from build123d import *

# Parameters (mm, degrees)
SKETCH_1_R          = 1
EXTRUDE_1_DEPTH     = 10.5
SKETCH_2_W          = 9.3
SKETCH_2_H          = 27
CUT_EXTRUDE_1_DEPTH = 10.5
FILLET_1_R          = 4
FILLET_2_R          = 0.3
SKETCH_3_R          = 1.25
CUT_EXTRUDE_2_DEPTH = 19


with BuildPart() as part:
    # 草图1 → 凸台-拉伸1 (new body)
    with BuildSketch(Plane.XY):
        with BuildLine():
            ThreePointArc((7, 0), (4, 3), (1, 0))
            Line((1, 0), (1, -1))
            Line((1, -1), (0, -1))
            Line((0, -1), (0, -21.5))
            add(Edge.make_bspline(
                [(0, -21.5), (0, -22.851375424), (-0.954237794, -23.948160578)],
                knots=[0, 0, 0, 0.976850958, 0.976850958, 0.976850958], degree=2))
            add(Edge.make_bspline(
                [(7, 0), (7, -3.461774358), (6.888539552, -11.820950193), (2.535059444, -19.986776398), (-0.954237794, -23.948160578)],
                knots=[0, 0, 0, 0, 0.379767853, 0.997303013, 0.997303013, 0.997303013, 0.997303013], degree=3))
        make_face()
        with Locations(Location((4, 0, 0), (0, 0, 180))):
            Circle(SKETCH_1_R, mode=Mode.SUBTRACT)
    extrude(amount=EXTRUDE_1_DEPTH)

    # 草图2 → 切除-拉伸1 (cut)
    with BuildSketch(Plane.ZY.offset(-0.6)):
        with Locations((5.25, -10.44816051)):
            Rectangle(SKETCH_2_W, SKETCH_2_H)
    extrude(amount=-CUT_EXTRUDE_1_DEPTH, mode=Mode.SUBTRACT)

    # 圆角1
    fillet_1_edges = [part.edges().sort_by_distance(p)[0] for p in [
        (0.6, -22.041590232, 5.25),
    ]]
    fillet(fillet_1_edges, radius=FILLET_1_R)

    # 圆角2
    fillet_2_edges = [part.edges().sort_by_distance(p)[0] for p in [
        (0, -11.25, 10.5),
        (-0.248254444, -22.812327553, 0),
        (0, -11.25, 0),
        (1, -1, 10.2),
        (-0.248254444, -22.812327553, 10.5),
        (1, -1, 0.3),
    ]]
    fillet(fillet_2_edges, radius=FILLET_2_R)

    # 草图3 → 切除-拉伸2 (cut)
    with BuildSketch(Plane(origin=(0, 0, 0), x_dir=(-1, 0, 0), z_dir=(0, 0, -1))):
        with Locations(Location((-3.2, -8.5, 0), (0, 0, 270))):
            Circle(SKETCH_3_R)
    extrude(amount=-CUT_EXTRUDE_2_DEPTH, mode=Mode.SUBTRACT)


solid = part.part
CAD build for the part. Positions are in the model's coordinates, mm. A direction names the side the tool comes from. Give positions to 0.01 mm unless a question says otherwise; leave off trailing zeros. Answer in a Markdown table with one row per item. Add a question column.
Item 1: Drop flat-ended pins along their axis: P1, Ø0.6, axis at x = 0, z = 7.5, coming from the +Y side; P2, Ø2, axis at x = 3.5, z = 5, coming from the -Y side; P3, Ø1, axis at y = -4.5, z = 8.5, coming from the -X side; P4, Ø3, axis at y = -13.5, z = 3.5, coming from the +X side. Give the stop position or say it passes through.
Item 2: Probe probe 1 along Z at (x, y) = (1.25, -2); probe 2 along Y at (x, z) = (4, 0.25); probe 3 along X at (y, z) = (-13, 2.75). List the from-to ranges inside material, lowest first.
Item 3: Tool access for faces 1 (the face through (0, -11, 5)), 2 (the face through (3, -7, 10.5)), 3 (the face through (0.6, -11, 5)): list every direction of +Z, -Z, +X, -X, +Y, -Y with a clear straight run to the whole face (end or side of a thin tool).
Item 4: Mould opens along Y. For faces 4 (the face through (4.1, 3, 0.3)), 5 (the face through (4, -7, 0.6)), 6 (the face through (4.8, 0.6, 0.3)) say: +Y half, -Y half, draft (parallel to the pull), parting line (faces both ways), or undercut.
Item 5: Band-saw the part on A-A on x = 3.75. Give the number of separate pieces and of enclosed holes in the cut face, then the cut area to 3 significant figures.
Reply:
| question | item | result |
|---|---|---|
| 1 | P1 | stops at y = -1 |
| 1 | P2 | passes through |
| 1 | P3 | stops at x = 0 |
| 1 | P4 | stops at x = 0.6 |
| 2 | probe 1 | z = 0 to 0.6, 9.9 to 10.5 |
| 2 | probe 2 | y = -16.47 to -9.46, -7.54 to -1, 1 to 3 |
| 2 | probe 3 | x = 0 to 0.6 |
| 3 | face 1 | +Z, -Z, -X, +Y |
| 3 | face 2 | +Z, +X, -X, +Y, -Y |
| 3 | face 3 | +X, +Y, -Y |
| 4 | face 4 | +Y half |
| 4 | face 5 | draft |
| 4 | face 6 | undercut |
| 5 | separate pieces | 6 |
| 5 | enclosed holes | 0 |
| 5 | area | 18.9 mm^2 |
